Autodesk Inventor part; units mm, degrees
ref_plane "YZ Plane" through (0, 0, 0) normal (1, 0, 0) x (0, 1, 0)
ref_plane "XZ Plane" through (0, 0, 0) normal (0, 1, 0) x (-1, 0, 0)
ref_plane "XY Plane" through (0, 0, 0) normal (0, 0, 1) x (1, 0, 0)
sketch "Sketch1" plane through (0, 0, 0) normal (0, 0, 1) x (1, 0, 0)
  line L0 (0, 0) -> (22.5, 0)
  line L1 (22.5, 0) -> (22.5, 23)
  line L2 (22.5, 23) -> (0, 23)
  line L3 (0, 23) -> (0, 0)
  dimension "d0" = 22.5
  dimension "d1" = 23
extrude "Extrusion1" add sketch "Sketch1" along normal blind 12.2
sketch "Sketch2" plane through (0, 0, 0) normal (0, -1, 0) x (1, 0, 0)
  line L0 (0, 12.2) -> (22.5, 12.2)
  line L1 (0, 0) -> (22.5, 0)
  line L2 (1.6, 12.2) -> (4.1, 12.2)
  line L3 (4.1, 12.2) -> (4.1, 0)
  line L4 (4.1, 0) -> (1.6, 0)
  line L5 (1.6, 0) -> (1.6, 12.2)
  line L6 (22.5, 0) -> (22.5, 12.2)
  dimension "d4" = 2.5
  dimension "d5" = 18.4
extrude "Extrusion2" add sketch "Sketch2" along normal blind 5 contours L0 L3 L1 L5
ref_plane "Work Plane1" through (22.5, 11.5, 0) normal (0, -1, 0) x (1, 0, 0)
mirror "Mirror1" about plane through (22.5, 11.5, 0) normal (0, -1, 0) of "Extrusion2"
ref_plane "Work Plane3" through (0, -2.5, 0) normal (0, -1, 0) x (1, 0, 0)
ref_plane "Work Plane4" through (0, 0, 6.1) normal (0, 0, 1) x (1, 0, 0)
hole "Hole1" at (1.6, -2.5, 6.1) direction (1, 0, 0) diameter 2 end through all
mirror "Mirror2" about plane through (22.5, 11.5, 0) normal (0, -1, 0) of "Hole1"
sketch "Sketch3" plane through (22.5, 0, 0) normal (0, -1, 0) x (1, 0, 0)
  line L0 (-4.7, 4.35) -> (-6, 4.35)
  line L1 (-6, 4.35) -> (-6, 7.85)
  line L2 (-6, 7.85) -> (-4.7, 7.85)
  line L3 (-4.7, 7.85) -> (-4.7, 4.35)
  line L4 (0, 12.2) -> (0, 0)
  line L5 (0, 0) -> (-18.4, 0)
  line L6 (-18.4, 12.2) -> (-18.4, 0)
  line L7 (-20.9, 12.2) -> (-18.4, 12.2)
  line L8 (-20.9, 0) -> (-20.9, 12.2)
  line L9 (-20.9, 0) -> (-22.5, 0)
  line L10 (-22.5, 0) -> (-22.5, 12.2)
  line L11 (-22.5, 12.2) -> (-20.9, 12.2)
  line L12 (-18.4, 12.2) -> (0, 12.2)
  line L13 (-18.4, 0) -> (-20.9, 0)
  line L14 (0, 12.2) -> (0, 0)
  line L15 (0, 0) -> (-18.4, 0)
  line L16 (-18.4, 12.2) -> (-18.4, 0)
  line L17 (-20.9, 12.2) -> (-18.4, 12.2)
  line L18 (-20.9, 0) -> (-20.9, 12.2)
  line L19 (-20.9, 0) -> (-22.5, 0)
  line L20 (-22.5, 0) -> (-22.5, 12.2)
  line L21 (-22.5, 12.2) -> (-20.9, 12.2)
  line L22 (-18.4, 12.2) -> (0, 12.2)
  line L23 (-18.4, 0) -> (-20.9, 0)
  line L24 (0, 12.2) -> (0, 0)
  line L25 (0, 0) -> (-18.4, 0)
  line L26 (-18.4, 12.2) -> (-18.4, 0)
  line L27 (-20.9, 12.2) -> (-18.4, 12.2)
  line L28 (-20.9, 0) -> (-20.9, 12.2)
  line L29 (-20.9, 0) -> (-22.5, 0)
  line L30 (-22.5, 0) -> (-22.5, 12.2)
  line L31 (-22.5, 12.2) -> (-20.9, 12.2)
  line L32 (-18.4, 12.2) -> (0, 12.2)
  line L33 (-18.4, 0) -> (-20.9, 0)
  line L34 (-27, 6.1) -> (4.5, 6.1)
  point P0 (-6, 6.1)
  dimension "d17" = 1.3
  dimension "d18" = 3.5
  dimension "d19" = 4.7
extrude "Extrusion3" add sketch "Sketch3" along normal blind 2 contours L0 L1 L34 L3 | L34 L1 L2 L3
sketch "Sketch4" plane through (0, 0, 0) normal (-1, 0, 0) x (0, 0, 1)
  line L0 (6.1, 34.6) -> (6.1, -11.6)
  circle A0 centre (6.1, 6.1) radius 6.1
  line L1 (0, 0) -> (0, 23)
  line L2 (0, 0) -> (12.2, 0)
extrude "Extrusion4" add sketch "Sketch4" along normal blind 5.8 contours A0 L0 | L0 A0
sketch "Sketch5" plane through (-5.8, 6.1, 6.1) normal (-1, 0, 0) x (0, 0, 1)
  circle A0 centre (0, 0) radius 2
  point P0 (-6.1, -6.1)
  dimension "d24" = 4
extrude "Extrusion5" add sketch "Sketch5" along normal blind 1
sketch "Sketch6" plane through (0, 23, 0) normal (-1, 0, 0) x (0, 0, 1)
  circle A0 centre (6.1, -16.9) radius 6.1
  arc A1 (12.2, -16.9) -> (0, -16.9) centre (6.1, -16.9) ccw
  circle A2 centre (6.1854, -10.8006) radius 2.5717
  point P0 (0, -23)
extrude "Extrusion6" add sketch "Sketch6" along normal up to surface (5.8 mm away) contours A2 A0 | A0 A2 picked at (5.289, -10.1215) picked at (6.9125, -11.6556)
ref_plane "Work Plane2" through (22.5, 11.5, 0) normal (0, -1, 0) x (1, 0, 0)
properties part number "servo_metal_600TVL"
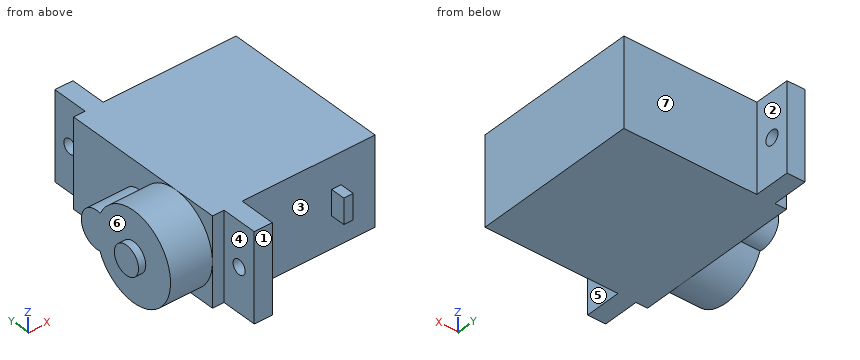
The listing builds one solid part. Answer for the finished solid, in the listing's coordinates (mm). Face numbers are marked on the shaded views. A direction names the side the tool comes from. Round coordinates to 2 decimals unless told otherwise and drop trailing zeros. Write each loop counter-clockwise with the first axis right and the second up, starting at its lowest first coordinate (ties: lowest second). Pieces come first, ordered by that corner, then holes. Notation, with made-up numbers: (-4, 5.5) -> (18, 5.5) arc R25 cw to (18, 33.5) -> close; hole circle Ø2 at (31.25, 24.5). An arc over 180 degrees is marked (long way). Use CSV: the item, a comma, the result in double quotes. Start each with the question number.
(1) Section D-D on z = 3 is taken. Give the vertices of the cut face in (x, y), then the cut area to 3 significant figures.
(2) Each of these flat-tipped pins is pushed along its axis until it touches: pin 1 (1 mm diameter, centred on x = 17, y = -1.5, fed in from -Z); pin 2 (1.6 mm diameter, centred on y = -1, z = 6.5, fed in from +X); pin 3 (2.5 mm diameter, centred on y = 25.5, z = 6.1, fed in from +X); pin 4 (4 mm diameter, centred on x = -2, y = 23.5, fed in from -Z). Where does it stop, or does it pass through?
(3) Section B-B on x = 3.5 is taken. Give the vertices of the cut face in (y, z).
(4) Which of the six approach directions +Z, -Z, +X, -X, +Y, -Y give full straight-line access (tool end or side, diameter ignored) to the marked faces 4, 5, 6 and 7?
(5) The mould has two halves that part along X. Classify the marked faces 1, 2 and 3: released by +X, released by -X, zero draft, split by the parting line, or undercut.
(6) Section A-A on y = -2.5 is taken. Give the vertices of the cut face in (x, z).
(7) Consider L1, parallel to Y at x = 3.1, z = 6.1; L2, parallel to Z at x = 2.4, y = 25.5; L3, parallel to Y at x = 16.75, z = 11.5. Determine where each line is inside the solid, lowest interval first. Write a range as from..to.
(8) Section C-C on z = 6.5 is taken. Count the separate pieces of the cut face and the enclosed holes in it, then the cut area to 3 significant figures.
A:
1,outline,"(-5.8, 0.85) -> (0, 0.85) -> (0, 0) -> (1.6, 0) -> (1.6, -5) -> (4.1, -5) -> (4.1, 0) -> (22.5, 0) -> (22.5, 23) -> (4.1, 23) -> (4.1, 28) -> (1.6, 28) -> (1.6, 23) -> (0, 23) -> (0, 11.35) -> (-5.8, 11.35) -> close"
1,area,"603 mm²"
2,pin 1,"stops at z = 4.35"
2,pin 2,"stops at x = 17.8"
2,pin 3,"stops at x = 4.1"
2,pin 4,"passes through"
3,outline,"(-5, 0) -> (28, 0) -> (28, 12.2) -> (-5, 12.2) -> close; hole circle Ø2 at (-2.5, 6.1); hole circle Ø2 at (25.5, 6.1)"
4,face 4,"+Z, -Z, -X, -Y"
4,face 5,"+Z, -Z, -Y"
4,face 6,"-X"
4,face 7,"+Z, -Z, +X, +Y"
5,face 1,"zero draft"
5,face 2,"released by +X"
5,face 3,"undercut"
6,outline,"(1.6, 0) -> (4.1, 0) -> (4.1, 5.1) -> (1.6, 5.1) -> close; (1.6, 7.1) -> (4.1, 7.1) -> (4.1, 12.2) -> (1.6, 12.2) -> close"
7,L1,"y = -5..-3.5, -1.5..24.5, 26.5..28"
7,L2,"z = 0..5.1, 7.1..12.2"
7,L3,"y = 0..23"
8,separate pieces,"3"
8,enclosed holes,"0"
8,area,"625 mm²"
